Check sheet for the drawn part. Datum: minimum x, y, z corner. Units: mm. Give positions to 0.01 mm unless a question says otherwise; leave off trailing zeros. Write each loop counter-clockwise with the first axis right and the second up, starting at its lowest first coordinate (ties: lowest second). Pieces come first, ordered by that corner, then holes. Notation, with made-up numbers: (4, 87.5) - (20, 87.5) arc R31 ccw to (20, 126.5) - close; hole circle Ø7 at (-26.5, 75.5). An arc over 180 degrees is marked (long way). Answer as a JSON object with one key per item and string values. Group by question number.
Item 1: Sectioned sample at C-C, the plane y = 6.75. Record the boundary of the cut face in (x, z), and give its area (3 significant figures).
Item 2: Sectioned sample at B-B, the plane x = 18.5. Record the boundary of the cut face in (y, z), and give its area (3 significant figures).
Item 3: Sectioned sample at D-D, the plane x = 28. Record the boundary of the cut face in (y, z) (1 decimal).
Item 4: Scan lines: line 1 along X through (y, z) = (6.5, 8.5) (1 decimal); line 2 along X through (y, z) = (10, 8.5) (1 decimal); line 3 along Z through (x, y) = (14, 11). Record each from-to range of solid material in increasing order. Write a range as [from, to].
Item 5: Draft check along X on the marked faces 1, 2, 3 and 4. Enter one of: +X half, -X half, draft (parallel to the pull), parting line (faces both ways), or undercut.
Item 6: Sectioned sample at A-A, the plane y = 10.75. Record the boundary of the cut face in (x, z) (1 decimal), and give its area (3 significant figures).
Item 7: Go/stop test with flat-tipped pins: pin 1 (1.3 mm diameter, centred on x = 20.5, y = 10.5, fed in from +Z); pin 2 (5 mm diameter, centred on x = 10.14, y = 7.38, fed in from +Z); pin 3 (1.5 mm diameter, centred on x = 28.49, y = 7.38, fed in from -Z). Record where each tip stops, or that it passes through.
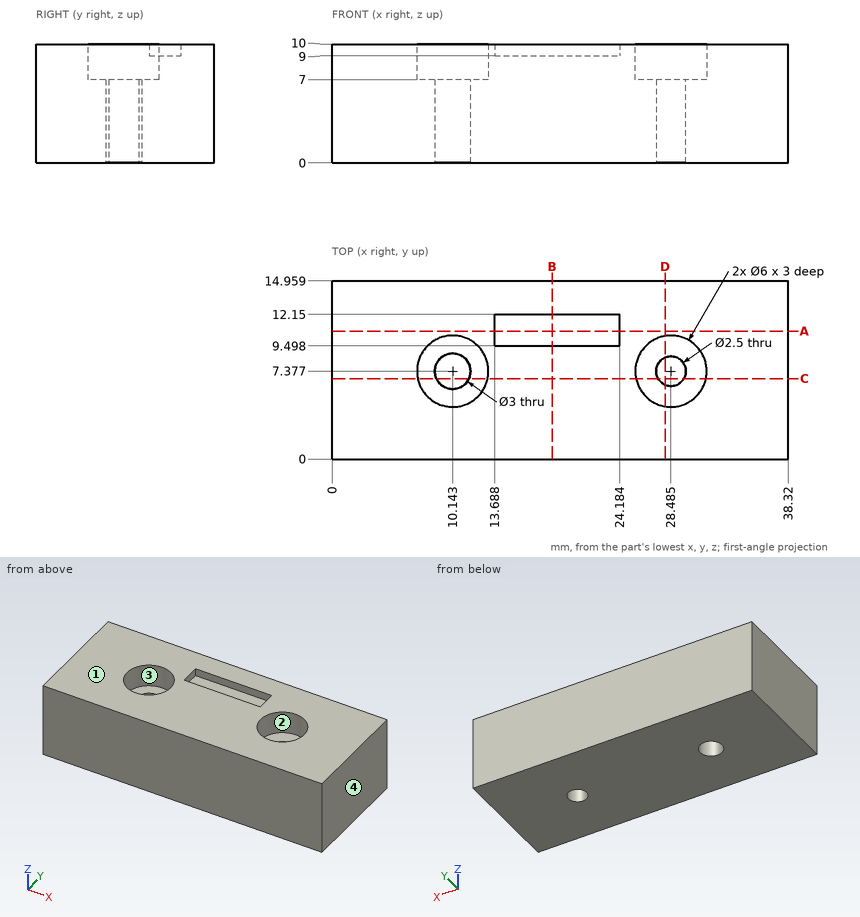
Geometry check:
{
 "1": {"outline": "(0, 0) - (8.78, 0) - (8.78, 7) - (7.21, 7) - (7.21, 10) - (0, 10) - close; (11.51, 0) - (27.4, 0) - (27.4, 7) - (25.55, 7) - (25.55, 10) - (13.08, 10) - (13.08, 7) - (11.51, 7) - close; (29.57, 0) - (38.32, 0) - (38.32, 10) - (31.42, 10) - (31.42, 7) - (29.57, 7) - close", "area": "314 mm^2"},
 "2": {"outline": "(0, 0) - (14.96, 0) - (14.96, 10) - (12.15, 10) - (12.15, 9) - (9.5, 9) - (9.5, 10) - (0, 10) - close", "area": "147 mm^2"},
 "3": {"outline": "(0, 0) - (6.2, 0) - (6.2, 7) - (4.4, 7) - (4.4, 10) - (0, 10) - close; (8.5, 0) - (15, 0) - (15, 10) - (10.3, 10) - (10.3, 7) - (8.5, 7) - close"},
 "4": {"line 1": "[0, 7.3], [13, 25.6], [31.4, 38.3]", "line 2": "[0, 8.7], [11.6, 27], [29.9, 38.3]", "line 3": "[0, 9]"},
 "5": {"face 1": "draft", "face 2": "undercut", "face 3": "undercut", "face 4": "+X half"},
 "6": {"outline": "(0, 0) - (38.3, 0) - (38.3, 10) - (24.2, 10) - (24.2, 9) - (13.7, 9) - (13.7, 10) - (0, 10) - close", "area": "373 mm^2"},
 "7": {"pin 1": "z = 9", "pin 2": "z = 7", "pin 3": "through"}
}
